```python
from build123d import *

# Parameters (mm, degrees)
F0_R      = 23.1963594976
F0_W      = 20.5508206286
F0_H      = 16.1379426718
F0_W_2    = 19.1440358758
F0_H_2    = 15.3468698263
F1_DEPTH  = 101.6
F3_DEPTH  = 152.4
F4_R      = 21.9223320718
F5_DEPTH  = 254
F6_W      = 70.3377723694
F6_H      = 45.2993959188
F7_DEPTH  = 25.4
F8_W      = 23.4599709511
F8_H      = 44.165968895
F9_DEPTH  = 254
F10_W     = 16.7544244835
F10_H     = 44.361397624
F11_DEPTH = 25


with BuildPart() as f1:
    # F0 (on Front) → F1 (new body)
    with BuildSketch(Plane.XZ):
        Polygon((40.1767790318, 53.0281364918), (-66.7938407264, 53.0281364918), (-66.7938407264, 36.89019382), (-17.7499198207, 36.89019382), (-17.7499198207, -32.2498530149), (-67.8841918707, -32.2498530149), (-67.8841918707, -47.5967228413), (37.6453399658, -47.5967228413), (76.091632247, -24.1808742285), (76.091632247, 27.0808488131), align=None)
        with Locations((39.0692800283, 0)):
            Circle(F0_R, mode=Mode.SUBTRACT)
        with Locations((-77.0692510407, 44.9591651559)):
            Rectangle(F0_W, F0_H)
        with Locations((-77.4562098086, -39.9232879281)):
            Rectangle(F0_W_2, F0_H_2)
    extrude(amount=F1_DEPTH)

    # F2 (on face) → F3 (cut)
    with BuildSketch(Plane.XY.offset(53.0281364918)):
        Polygon((-87.344661355, 0), (-87.344661355, -22.4940739572), (-66.105723381, 0), align=None)
        Polygon((-63.0609244108, -101.6), (-87.344661355, -82.5703293085), (-87.344661355, -101.6), align=None)
    extrude(amount=-F3_DEPTH, mode=Mode.SUBTRACT)

    # F4 (on face) → F5 (cut)
    with BuildSketch(Plane.XY.offset(53.0281364918)):
        with Locations((-49.0250661969, -48.2343658805)):
            Circle(F4_R)
    extrude(amount=-F5_DEPTH, mode=Mode.SUBTRACT)

    # F6 (on face) → F7 (cut)
    with BuildSketch(Plane(origin=(38.9509155446, 0, 53.9137821149), x_dir=(0.810585134, 0, -0.5856208164), z_dir=(0.5856208164, 0, 0.810585134))):
        with Locations((21.9143256545, -49.9939098954)):
            Rectangle(F6_W, F6_H)
    extrude(amount=-F7_DEPTH, mode=Mode.SUBTRACT)

    # F8 (on face) → F9 (cut)
    with BuildSketch(Plane(origin=(0, 0, -47.5967228413), x_dir=(1, 0, 0), z_dir=(0, 0, -1))):
        with Locations((25.9153544903, 49.6352612972)):
            Rectangle(F8_W, F8_H)
    extrude(amount=-F9_DEPTH, mode=Mode.SUBTRACT)

    # F10 (on face) → F11 (cut)
    with BuildSketch(Plane(origin=(31.3311681007, 0, -51.4423912721), x_dir=(0.8540627897, 0, 0.5201699254), z_dir=(0.5201699254, 0, -0.8540627897))):
        with Locations((60.7860804046, 49.5375469327)):
            Rectangle(F10_W, F10_H)
    extrude(amount=-F11_DEPTH, mode=Mode.SUBTRACT)


solid = f1.part
```
The model under review builds one solid part; all positions refer to its coordinate system, in mm. A direction names the side the tool comes from. Round coordinates to 2 decimals unless told otherwise and drop trailing zeros. Order: outer loops, then holes, each group sorted by start corner. A loop starts at its lowest first (then second) coordinate and runs counter-clockwise, first axis right, second up.
(1) Take a section at D-D, the plane x = -51.5. State the section outline as (y, z) points, plus the area to 3 significant figures.
Working result:
outline: (-101.6, -47.6) - (-70.02, -47.6) - (-70.02, -32.25) - (-101.6, -32.25) - close; (-101.6, 36.89) - (-70.02, 36.89) - (-70.02, 53.03) - (-101.6, 53.03) - close; (-26.45, -47.6) - (0, -47.6) - (0, -32.25) - (-26.45, -32.25) - close; (-26.45, 36.89) - (0, 36.89) - (0, 53.03) - (-26.45, 53.03) - close
area: 1,830 mm2
(2) Take a section at A-A, the plane y = -24.5. State the section outline as (x, z) points.
Working result:
outline: (-87.34, 36.89) - (-17.75, 36.89) - (-17.75, -32.25) - (-87.03, -32.25) - (-87.03, -47.6) - (37.65, -47.6) - (76.09, -24.18) - (76.09, 27.08) - (40.18, 53.03) - (-87.34, 53.03) - close; hole circle Ø46.39 at (39.07, 0)
(3) Take a section at C-C, the plane z = -8.5. State the section outline as (x, y) points.
Working result:
outline: (-17.75, -101.6) - (17.49, -101.6) - (17.49, -71.72) - (14.19, -71.72) - (14.19, -27.55) - (17.49, -27.55) - (17.49, 0) - (-17.75, 0) - close; (60.65, -101.6) - (76.09, -101.6) - (76.09, -71.72) - (66.54, -71.72) - (66.54, -27.36) - (76.09, -27.36) - (76.09, 0) - (60.65, 0) - close
(4) Wall thickness on L1, parallel to Z at x = -65, y = -96.5; L2, parallel to X at y = -22, z = 0; L3, parallel to Y at x = 16, z = 34: over which ranges is each line inside the solid? List them lowest first.
Working result:
L1: z = -47.6 to -32.25, 36.89 to 53.03
L2: x = -17.75 to 15.87, 62.27 to 76.09
L3: y = -101.6 to -71.72, -27.55 to 0
(5) Tool access review of faces 4 (the face through (70, -71.718, -7)), 5 (the face through (-67.3, -61.4, -32.25)), 6 (the face through (16, -71.718, 50)), 7 (the face through (4, 0, 3)), 8 (the face through (58.39, -86.92, 39.87)): name each direction out of +Z, -Z, +X, -X, +Y, -Y from which nothing blocks a thin tool from reaching the whole face with its end or side.
Working result:
face 4: +X
face 5: -X, +Y, -Y
face 6: +Z, -Z, +X
face 7: +Z, -Z, +X, -X, +Y
face 8: +Z, +X, +Y, -Y
(6) Mouldability with a two-part tool opening along Z and no side actions: class faces 1 (the face through (66.04, -49.85, -1.03)), 2 (the face through (58.39, -13.48, 39.87)), 3 (the face through (-70.926, -47.27, 45.072)) as released by +Z, released by -Z, zero draft, split by the parting line, or undercut.
Working result:
face 1: undercut
face 2: released by +Z
face 3: zero draft
(7) Take a section at B-B, the plane y = -51. Count the separate pieces of the cut face and the enclosed holes in it, plus the area to 3 significant figures.
Working result:
separate pieces: 6
enclosed holes: 0
area: 4,810 mm2
(8) For P1, Ø5, axis at y = -20, z = -28.5, coming from the +X side; P2, Ø1.5, axis at y = -70, z = 35.5, coming from the -X side; P3, Ø4.5, axis at y = -42.5, z = -36.5, coming from the -X side, all flat-tipped, find the tip position at first contact; note any pin that passes through.
Working result:
P1: stops at x = 73.1
P2: stops at x = -17.75
P3: stops at x = -87.03
